The listing builds one solid part. Answer for the finished solid, in the listing's coordinates (mm). A direction names the side the tool comes from. Round coordinates to 2 decimals unless told otherwise and drop trailing zeros. Write each loop counter-clockwise with the first axis right and the second up, starting at its lowest first coordinate (ties: lowest second). Pieces come first, ordered by that corner, then holes.
Item 1: Find the intervals of material crossed by probe 1 along Y at (x, z) = (324, -31.5); probe 2 along Z at (x, y) = (694, 35); probe 3 along Y at (x, z) = (394, -140.5), in increasing order.
Item 2: A tool of negligible diameter and unlimited length cuts with its end or side. For faces 4 (the face through (519, 140, -74)), 5 (the face through (515, 150, -76)), from which of +Z, -Z, +X, -X, +Y, -Y can it reach the whole face along a straight path? Write none if from no direction.
Item 3: Find section D-D on x = 1080. Give the vertices of the cut face in (y, z), then the cut area to 3 significant figures.
Item 4: Find section B-B on x = 958. Give the vertices of the cut face in (y, z).
Item 5: For a pull along Z with two mould halves and no side action, classify faces 1 (the face through (576, 0, -74)), 2 (the face through (572, 76, 0)), 3 (the face through (572, 74, -140)) as +Z half, -Z half, draft (parallel to the pull), parting line (faces both ways), or undercut.
Item 6: Find section C-C on y = 82. Give the vertices of the cut face in (x, z), then the cut area to 3 significant figures.
Item 7: Find section A-A on z = -63.5. Give the vertices of the cut face in (x, y), then the cut area to 3 significant figures.
```python
from build123d import *

# Parameters (mm, degrees)
SKETCH1_W               = 130
SKETCH1_H               = 130
EXTRUDE1_DEPTH          = 1168
CUT_EXTRUDE1_DEPTH      = 1188.107408788
CUT_EXTRUDE1_DEPTH_BACK = 1188.107408788
CUT_EXTRUDE2_DEPTH      = 1188.107408788
CUT_EXTRUDE2_DEPTH_BACK = 1188.107408788


with BuildPart() as part:
    # Sketch1 → Extrude1 (new body)
    with BuildSketch(Plane(origin=(0, 0, 0), x_dir=(0, 0, -1), z_dir=(1, 0, 0))):
        with BuildLine():
            Line((10, 0), (140, 0))
            ThreePointArc((140, 0), (147.071067812, 2.928932188), (150, 10))
            Line((150, 10), (150, 140))
            ThreePointArc((150, 140), (147.071067812, 147.071067812), (140, 150))
            Line((140, 150), (10, 150))
            ThreePointArc((10, 150), (2.928932188, 147.071067812), (0, 140))
            Line((0, 140), (0, 10))
            ThreePointArc((0, 10), (2.928932188, 2.928932188), (10, 0))
        make_face()
        with Locations((75, 75)):
            Rectangle(SKETCH1_W, SKETCH1_H, mode=Mode.SUBTRACT)
    extrude(amount=EXTRUDE1_DEPTH)

    # Sketch2 → Cut-Extrude1 (cut, two sides: drawn at the far end of the back side and taken through both)
    with BuildSketch(Plane.XY.offset(-CUT_EXTRUDE1_DEPTH_BACK)):
        Polygon((2979.836763712, -1520.311560184), (1168, 0), (989.236961111, 150), (-822.599802601, 1670.311560184), (2218.023317767, 5293.985087608), (6020.459884081, 2103.36196724), align=None)
    extrude(amount=CUT_EXTRUDE1_DEPTH + CUT_EXTRUDE1_DEPTH_BACK, mode=Mode.SUBTRACT)

    # Sketch3 → Cut-Extrude2 (cut, two sides: drawn at the far end of the back side and taken through both)
    with BuildSketch(Plane.XY.offset(-CUT_EXTRUDE2_DEPTH_BACK)):
        Polygon((-808.940884793, -2222.546814643), (0, 0), (54.59553514, 150), (863.536419933, 2372.546814643), (-3581.557209352, 3990.428584229), (-5254.034514079, -604.665045056), align=None)
    extrude(amount=CUT_EXTRUDE2_DEPTH + CUT_EXTRUDE2_DEPTH_BACK, mode=Mode.SUBTRACT)


solid = part.part
```
Check values:
1. probe 1: y = 0 to 10, 140 to 150
1. probe 2: z = -150 to -140, -10 to 0
1. probe 3: y = 0.01 to 149.99
2. face 4: +X, -X
2. face 5: +Z, -Z, +X, -X, +Y
3. outline: (0, -140) arc R10 ccw to (10, -150) - (73.84, -150) - (73.84, -140) - (10, -140) - (10, -10) - (73.84, -10) - (73.84, 0) - (10, 0) arc R10 ccw to (0, -10) - close
3. area: 2,730 mm2
4. outline: (0, -140) arc R10 ccw to (10, -150) - (140, -150) arc R10 ccw to (150, -140) - (150, -10) arc R10 ccw to (140, 0) - (10, 0) arc R10 ccw to (0, -10) - close; hole (10, -140) - (140, -140) - (140, -10) - (10, -10) - close
5. face 1: draft
5. face 2: +Z half
5. face 3: undercut
6. outline: (29.85, -150) - (1070.28, -150) - (1070.28, -140) - (29.85, -140) - close; (29.85, -10) - (1070.28, -10) - (1070.28, 0) - (29.85, 0) - close
6. area: 20,800 mm2
7. outline: (0, 0) - (1168, 0) - (1156.08, 10) - (3.64, 10) - close; (50.96, 140) - (1001.15, 140) - (989.24, 150) - (54.6, 150) - close
7. area: 21,000 mm2
